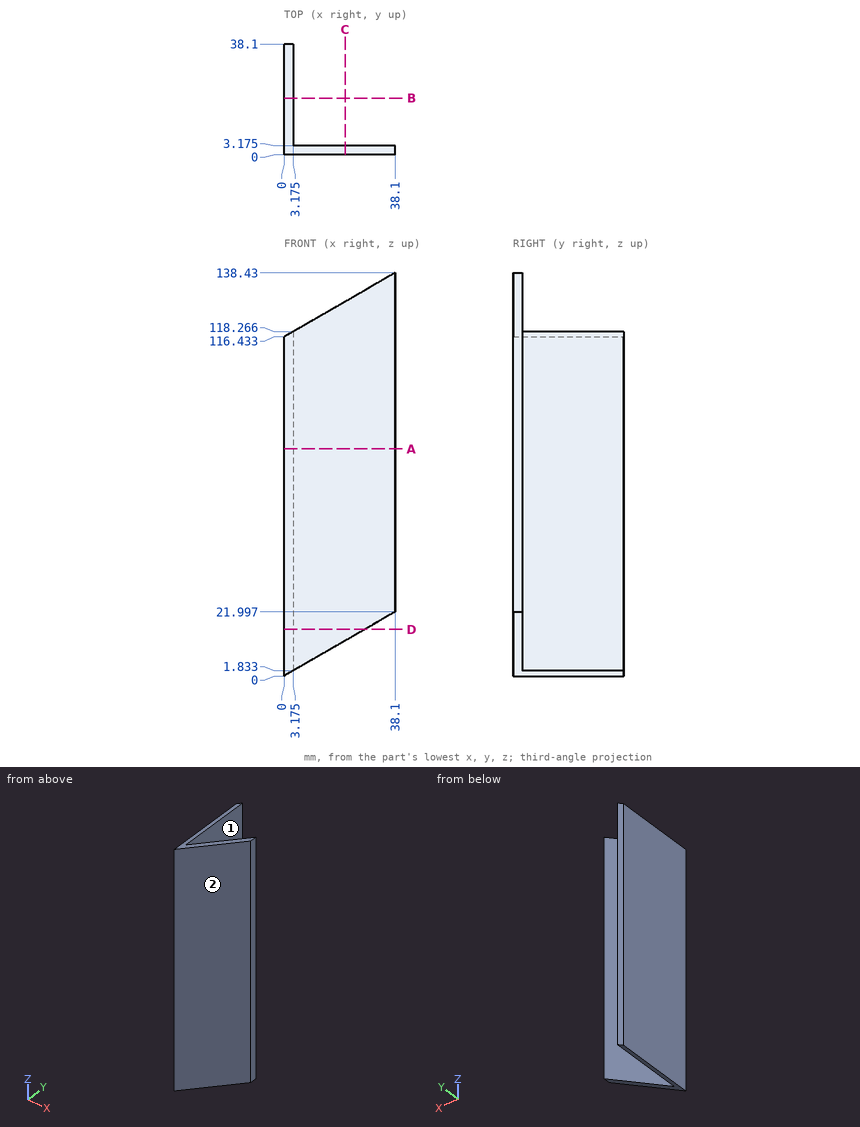
Job drawing, mm, ordinate dimensions from the low corner. One solid piece. A direction names the side the tool comes from. Give positions to 0.01 mm unless a question says otherwise; leave off trailing zeros. Write each loop counter-clockwise with the first axis right and the second up, starting at its lowest first coordinate (ties: lowest second). Pieces come first, ordered by that corner, then holes. Notation, with made-up numbers: M -9,31 L 29,31 A22 cw 29,65 Z; hole C 85.25,-16.75 d1. An arc over 180 degrees is marked long. Put each result on its own line as item: value. Start each with the question number.
(1) Band-saw the part on A-A, the plane z = 78. Write the cut outline in (x, y) (3 decimals), and give its area (3 significant figures).
(2) Band-saw the part on C-C, the plane x = 21. Write the cut outline in (y, z) (1 decimal), and give its area (3 significant figures).
(3) Which spindle directions (+Z, -Z, +X, -X, +Y, -Y) get a long thin tool onto all of the face, cutting with end or side? Do the marked faces 1 and 2. Say none if no direction does.
(4) Band-saw the part on D-D, the plane z = 16. Write the cut outline in (x, y) (3 decimals).
(5) Flat gauge pins, fed straight in: pin 1 Ø12 at (x, z) = (13.5, 24.5) entering from +Y (3 decimals); pin 2 Ø6 at (y, z) = (16.5, 89) entering from +X (3 decimals). Where does each tip first touch, or does it go through?
(6) Probe L1, parallel to X at y = 22.5, z = 18 (3 decimals); L2, parallel to Z at x = 25, y = 2.5. List the from-to ranges inside material, lowest first.
(7) Band-saw the part on B-B, the plane y = 19.5. Write the cut outline in (x, z) (3 decimals), and give its area (3 significant figures).
Response values:
1. outline: M 0,0 L 38.1,0 L 38.1,3.175 L 3.175,3.175 L 3.175,38.1 L 0,38.1 Z
1. area: 232 mm2
2. outline: M 0,12.1 L 3.2,12.1 L 3.2,128.6 L 0,128.6 Z
2. area: 370 mm2
3. face 1: +Z, -Z, +X, +Y
3. face 2: +Z, -Z, +X, -X, -Y
4. outline: M 0,0 L 27.713,0 L 27.713,3.175 L 3.175,3.175 L 3.175,38.1 L 0,38.1 Z
5. pin 1: stops at y = 3.175
5. pin 2: stops at x = 3.175
6. L1: x = 0 to 3.175
6. L2: z = 14.43 to 130.87
7. outline: M 0,0 L 3.175,1.833 L 3.175,118.266 L 0,116.433 Z
7. area: 370 mm2
